```python
from build123d import *

# Parameters (mm, degrees)
SKETCH1_R           = 1.85
BOSS_EXTRUDE1_DEPTH = 3.1
SKETCH2_R           = 1.5
BOSS_EXTRUDE2_DEPTH = 1
SKETCH3_R           = 1.1
BOSS_EXTRUDE3_DEPTH = 2
SKETCH6_W           = 5
SKETCH6_H           = 5
BOSS_EXTRUDE4_DEPTH = 5
SKETCH7_R           = 0.9
CUT_EXTRUDE1_DEPTH  = 3


with BuildPart() as part:
    # Sketch1 → Boss-Extrude1 (new body)
    with BuildSketch(Plane(origin=(0, 0, 0), x_dir=(1, 0, 0), z_dir=(0, 1, 0))):
        with Locations(Location((0, 0, 0), (0, 0, 90))):
            Circle(SKETCH1_R)
    extrude(amount=BOSS_EXTRUDE1_DEPTH)

    # Sketch2 → Boss-Extrude2 (add)
    with BuildSketch(Plane(origin=(0, 3.1, 0), x_dir=(1, 0, 0), z_dir=(0, 1, 0))):
        with Locations(Location((0, 0, 0), (0, 0, 270))):
            Circle(SKETCH2_R)
    extrude(amount=BOSS_EXTRUDE2_DEPTH)

    # Sketch3 → Boss-Extrude3 (add)
    with BuildSketch(Plane(origin=(0, 4.1, 0), x_dir=(1, 0, 0), z_dir=(0, 1, 0))):
        with Locations(Location((0, 0, 0), (0, 0, 270))):
            Circle(SKETCH3_R)
    extrude(amount=BOSS_EXTRUDE3_DEPTH)

    # Loft1: read off the stored shape, not the designer's step
    # Loft1: loft between two sections, ruled curve by curve
    loft1_from = [
        Edge.make_bspline([(0, 6.1, 1.85), (3.7, 6.1, 1.85), (3.7, 6.1, -1.85), (0, 6.1, -1.85), (-3.7, 6.1, -1.85), (-3.7, 6.1, 1.85), (0, 6.1, 1.85)], [0, 0, 0, 0, 0.5, 0.5, 0.5, 1, 1, 1, 1], 3, [1, 0.333333333, 0.333333333, 1, 0.333333333, 0.333333333, 1]),
    ]
    loft1_to = [
        Edge.make_bspline([(0.620465421, 8.6, 0.968257539), (2.556980499, 8.6, -0.272673303), (1.316049657, 8.6, -2.209188381), (-0.620465421, 8.6, -0.968257539), (-2.556980499, 8.6, 0.272673303), (-1.316049657, 8.6, 2.209188381), (0.620465421, 8.6, 0.968257539)], [0, 0, 0, 0, 0.5, 0.5, 0.5, 1, 1, 1, 1], 3, [1, 0.333333333, 0.333333333, 1, 0.333333333, 0.333333333, 1]),
    ]
    loft1 = Solid(Shell([*[Face.make_surface_from_curves(loft1_from[k], loft1_to[k]) for k in range(1)], Face(Wire(loft1_from)), Face(Wire(loft1_to))]))
    add(loft1)

    # Sketch6 → Boss-Extrude4 (add)
    with BuildSketch(Plane.XZ):
        Rectangle(SKETCH6_W, SKETCH6_H)
    extrude(amount=BOSS_EXTRUDE4_DEPTH)

    # Sketch7 → Cut-Extrude1 (cut)
    with BuildSketch(Plane.XZ.offset(5)):
        with Locations(Location((0, 0, 0), (0, 0, 270))):
            Circle(SKETCH7_R)
    extrude(amount=-CUT_EXTRUDE1_DEPTH, mode=Mode.SUBTRACT)


solid = part.part
```
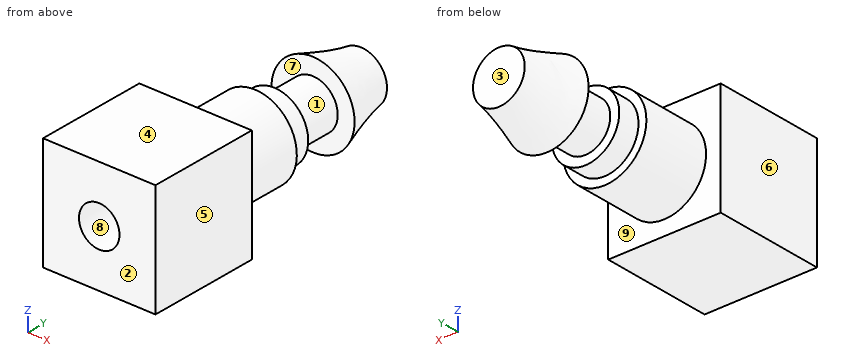
CAD build for the part. Positions are in the model's coordinates, mm. Face numbers are marked on the shaded views. A direction names the side the tool comes from. Round coordinates to 2 decimals unless told otherwise and drop trailing zeros. Write each loop counter-clockwise with the first axis right and the second up, starting at its lowest first coordinate (ties: lowest second). Pieces come first, ordered by that corner, then holes.
Item 1: Band-saw the part on C-C on y = 1.5. Write the cut outline in (x, z), then the cut area to 3 significant figures.
Filled in:
outline: circle Ø3.7 at (0, 0)
area: 10.8 mm2
Item 2: Tool access for the marked faces 5, 6, 7, 8 and 9: list every direction of +Z, -Z, +X, -X, +Y, -Y with a clear straight run to the whole face (end or side of a thin tool).
Filled in:
face 5: +Z, -Z, +X, +Y, -Y
face 6: +Z, -Z, -X, +Y, -Y
face 7: none
face 8: -Y
face 9: +Y
Item 3: Mould opens along Y. For the marked faces 1, 2, 3 and 4 say: released by +Y, released by -Y, zero draft, split by the parting line, or undercut.
Filled in:
face 1: undercut
face 2: released by -Y
face 3: released by +Y
face 4: zero draft
Item 4: Band-saw the part on B-B on y = 3.5. Write the cut outline in (x, z), then the cut area to 3 significant figures.
Filled in:
outline: circle Ø3 at (0, 0)
area: 7.07 mm2
Item 5: Band-saw the part on A-A on y = -4. Write the cut outline in (x, z), then the cut area to 3 significant figures.
Filled in:
outline: (-2.5, -2.5) - (2.5, -2.5) - (2.5, 2.5) - (-2.5, 2.5) - close; hole circle Ø1.8 at (0, 0)
area: 22.5 mm2
Item 6: Drill centre lines: L1, parallel to X at y = -4.3, z = 0; L2, parallel to Y at x = -1.95, z = -0.25; L3, parallel to X at y = 3.5, z = 0.1. Where is each one in solid material? Low to high.
Filled in:
L1: x = -2.5 to -0.9, 0.9 to 2.5
L2: y = -5 to 0
L3: x = -1.5 to 1.5
